Here's the drawing with two shaded views (mm, measured from the low corner). I have some questions. Give positions to 0.01 mm unless a question says otherwise; leave off trailing zeros. Loops run counter-clockwise (first coordinate to the right, second up) from the corner with the lowest first, then second, coordinate; pieces in that order, holes last. Notation, with made-up numbers: M 53,-22.75 L 89,-22.75 A38 ccw 89,15.25 Z; hole C -14,28.25 d5. An arc over 180 degrees is marked long. Write item = value, one per line. Start each with the question number.
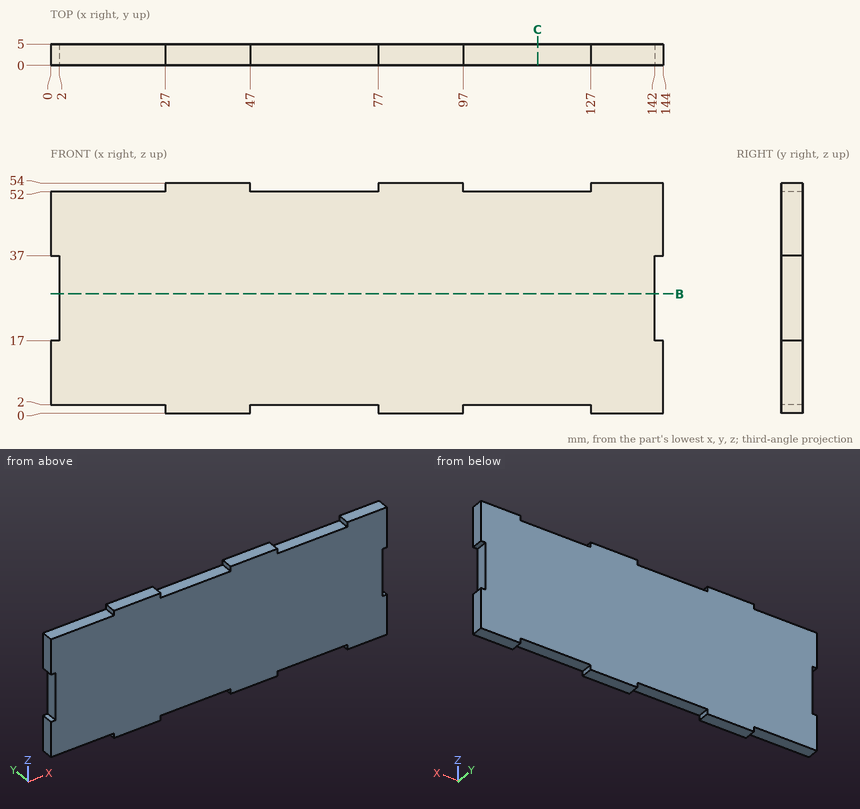
Q1. If we section it at B-B, the plane z = 28: List the corners of the cut face in (x, y) for me, then the cut area to 3 significant figures.
Q2. Will these pins go through, and if not, where does the flat tip stop? pin 1 (2 mm diameter, centred on y = 0.5, z = 30.5, fed in from +X); pin 2 (1.5 mm diameter, centred on x = 118, y = 3, fed in from -Z); pin 3 (1 mm diameter, centred on y = 3.5, z = 1, fed in from -X).
Q3. If I drill on line 1 along X through (y, z) = (0.35, 32); line 2 along Z through (x, y) = (125, 2.9), over which ranges is the centre line in solid material (lowest first)?
Q4. If we section it at C-C, the plane x = 114.5: List the corners of the cut face in (y, z) for me.
Resolved:
q1.outline = M 2,0 L 142,0 L 142,5 L 2,5 Z
q1.area = 700 mm²
q2.pin_1 = 142
q2.pin_2 = 2
q2.pin_3 = 27
q3.line_1 = 2 to 142
q3.line_2 = 2 to 52
q4.outline = M 0,2 L 5,2 L 5,52 L 0,52 Z
